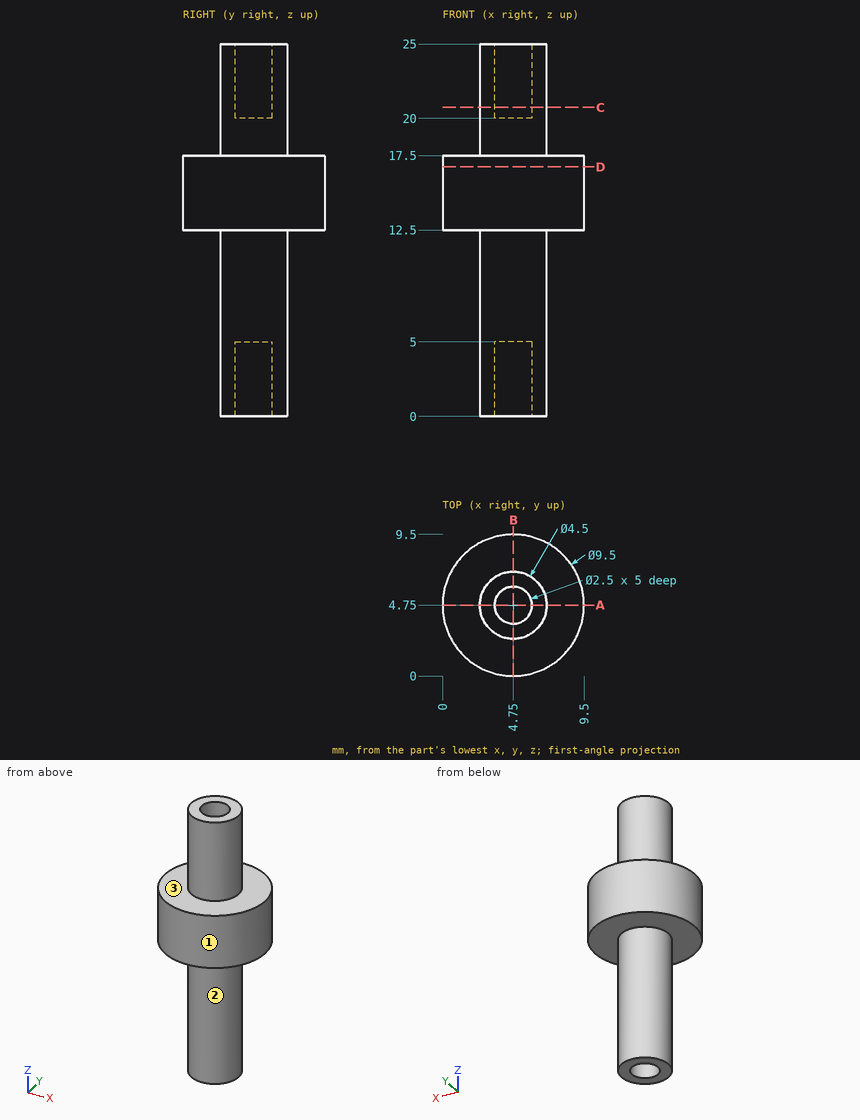
Study the drawing (mm; zero at the part's minimum x, y, z) and answer. A direction names the side the tool comes from. Round coordinates to 2 decimals unless told otherwise and drop trailing zeros. Order: outer loops, then holes, each group sorted by start corner. A loop starts at its lowest first (then second) coordinate and runs counter-clockwise, first axis right, second up. Notation, with made-up numbers: M 54,82 L 76,82 A22 cw 76,115 Z; hole C 14.25,53 d6. An arc over 180 degrees is marked long. One line per item, written item: value.
Q1. Straight lines are drawn through the part: line 1 (Y direction, x = 4.75, z = 3.2); line 2 (Z direction, x = 2.75, y = 7.5). For each, find the intervals that lie inside material, in ascending order.
Derived:
line 1: 2.5 to 3.5, 6 to 7
line 2: 12.5 to 17.5
Q2. Flat-ended cylindrical pins translate along their axes: pin 1 (1 mm diameter, centred on x = 1, y = 5, fed in from +Z); pin 2 (2 mm diameter, centred on x = 4.75, y = 4.75, fed in from -Z); pin 3 (4 mm diameter, centred on x = 7, z = 9, fed in from -Y). Find the tip coordinate at first contact, or state that the pin passes through.
Derived:
pin 1: z = 17.5
pin 2: z = 5
pin 3: y = 2.51
Q3. Find section A-A on y = 4.75. Write down the section's boundary in (x, z), then the cut area to 4 significant figures.
Derived:
outline: M 0,12.5 L 2.5,12.5 L 2.5,0 L 3.5,0 L 3.5,5 L 6,5 L 6,0 L 7,0 L 7,12.5 L 9.5,12.5 L 9.5,17.5 L 7,17.5 L 7,25 L 6,25 L 6,20 L 3.5,20 L 3.5,25 L 2.5,25 L 2.5,17.5 L 0,17.5 Z
area: 112.5 mm²
Q4. For the marked faces 1, 2 and 3, determine the directions among +Z, -Z, +X, -X, +Y, -Y from which every point of the face is accessible in a straight line to the end or side of a thin tool.
Derived:
face 1: +Z, -Z
face 2: -Z
face 3: +Z
Q5. Find section C-C on z = 20.75. Write down the section's boundary in (x, y), then the cut area to 3 significant figures.
Derived:
outline: C 4.75,4.75 d4.5; hole C 4.75,4.75 d2.5
area: 11.0 mm²
Q6. Find section D-D on z = 16.75. Write down the section's boundary in (x, y).
Derived:
outline: C 4.75,4.75 d9.5
